```python
from build123d import *


with BuildPart() as part:
    # Sketch1 → Revolve1 (revolve)
    with BuildSketch(Plane(origin=(0, 0, 0), x_dir=(0, 0, -1), z_dir=(1, 0, 0)), mode=Mode.PRIVATE) as revolve1_sk:
        with BuildLine():
            Line((9.271, 8.3312), (9.525, 8.5852))
            Line((9.525, 8.5852), (9.525, 9.109220524))
            ThreePointArc((9.525, 9.109220524), (6.878832982, 12.796695255), (3.430721893, 15.748))
            Line((3.430721893, 15.748), (0.762, 15.748))
            ThreePointArc((0.762, 15.748), (0.223184633, 15.524815367), (0, 14.986))
            Line((0, 14.986), (0, 8.5852))
            Line((0, 8.5852), (0.254, 8.3312))
            Line((0.254, 8.3312), (9.271, 8.3312))
        make_face()
    revolve(revolve1_sk.sketch.rotate(Axis((0, 0, -32.643147388), (0, 0, -1)), 90), axis=Axis((0, 0, -32.643147388), (0, 0, -1)))


solid = part.part
```
CAD build for the part. Positions are in the model's coordinates, mm. Coordinates: 2 decimals unless noted, no trailing zeros. Loops run counter-clockwise (first coordinate to the right, second up) from the corner with the lowest first, then second, coordinate; pieces in that order, holes last. Notation, with made-up numbers: (6, 81.25) - (34, 81.25) arc R6 ccw to (34, 85.25) - close; hole circle Ø10 at (8.5, 8). An arc over 180 degrees is marked (long way). Use CSV: the item, a comma, the result in double quotes. Start each with the question number.
Q1. Drop flat-ended pins along their axis: P1, Ø3, axis at x = 3, y = -12, coming from the -Z side; P2, Ø3, axis at x = 4.5, z = -3, coming from the +Y side; P3, Ø12, axis at x = -7.5, y = 0, coming from the +Z side; P4, Ø1, axis at x = 2.5, z = -2, coming from the +Y side. Give the stop position or say it passes through.
Q2. Cut at A-A, the plane x = 0. List the corners of the cut face in (y, z) (3 decimals), then the cut area to 3 significant figures.
Q3. Two-plate mould, pull along Y, no slides. Class faces 1 (the flat face through (6.5, 6.5, 0)), 2 (the cylindrical face through (7.946, -2.502, -4.826)), 3 (the cylindrical face through (7.27, 13.97, -2.08)): +Y half, -Y half, draft (parallel to the pull), parting line (faces both ways), or undercut.
Q4. Probe probe 1 along Y at (x, z) = (0, -4.5); probe 2 along Y at (x, z) = (2, -7.5); probe 3 along X at (y, z) = (5, -1.5). List the from-to ranges inside material, lowest first. Write a range as from..to.
Q5. Cut at C-C, the plane z = -7.25. List the corners of the cut face in (x, y), then the cut area to 3 significant figures.
Here are the results:
1,P1,"z = -8.43"
1,P2,"y = 15.46"
1,P3,"z = 0"
1,P4,"y = 15.62"
2,outline,"(-15.748, -3.431) arc R18.923 ccw to (-9.109, -9.525) - (-8.585, -9.525) - (-8.331, -9.271) - (-8.331, -0.254) - (-8.585, 0) - (-14.986, 0) arc R0.762 ccw to (-15.748, -0.762) - close; (8.331, -9.271) - (8.585, -9.525) - (9.109, -9.525) arc R18.923 ccw to (15.748, -3.431) - (15.748, -0.762) arc R0.762 ccw to (14.986, 0) - (8.585, 0) - (8.331, -0.254) - close"
2,area,"107 mm2"
3,face 1,"draft"
3,face 2,"undercut"
3,face 3,"parting line"
4,probe 1,"-14.98..-8.33, 8.33..14.98"
4,probe 2,"-11.92..-8.09, 8.09..11.92"
4,probe 3,"-14.93..-6.66, 6.66..14.93"
5,outline,"circle Ø24.76 at (0, 0); hole circle Ø16.66 at (0, 0)"
5,area,"263 mm2"
